Can you work these out from the drawing? Everything is in mm from the part's minimum corner. A direction names the side the tool comes from. Coordinates: 2 decimals unless noted, no trailing zeros. Loops run counter-clockwise (first coordinate to the right, second up) from the corner with the lowest first, then second, coordinate; pieces in that order, holes last. Notation, with made-up numbers: (31, 34) -> (50, 34) arc R22 ccw to (50, 66) -> close; hole circle Ø9 at (21, 88.25). An arc over 180 degrees is marked (long way). One line per question, with ' | ' between items.
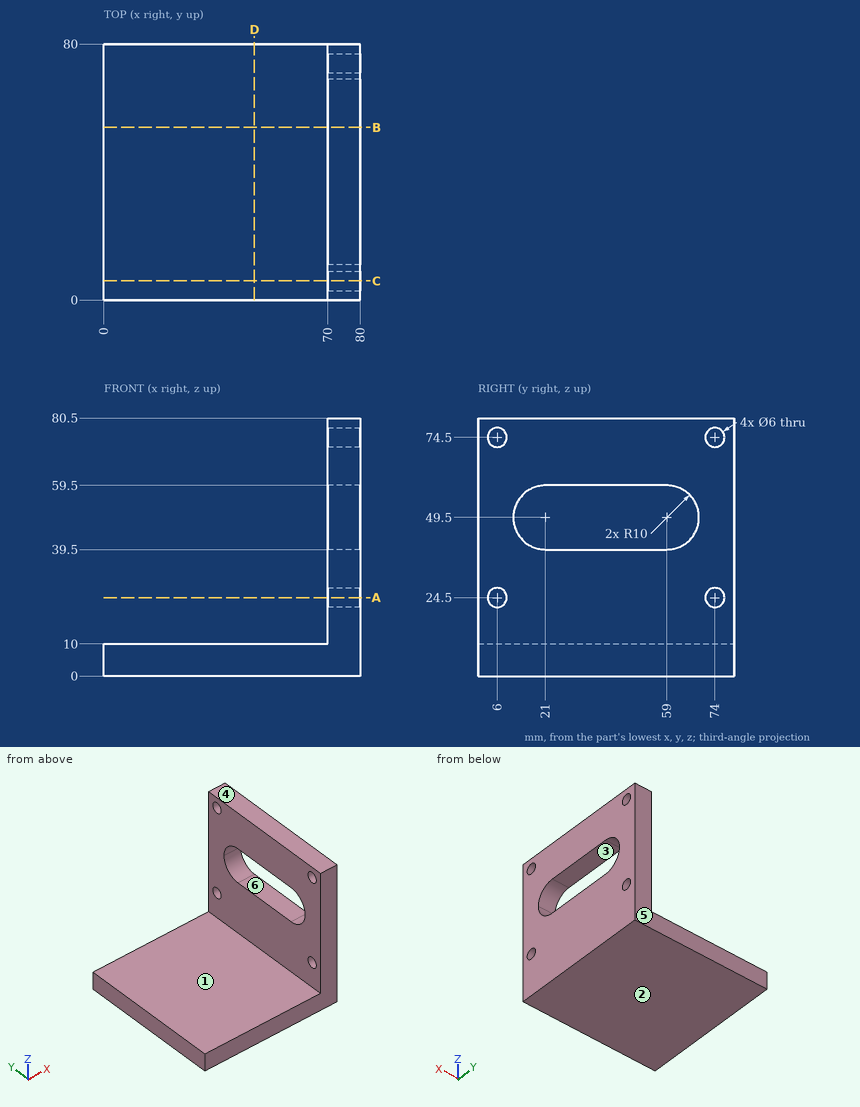
Q1. Please list where these lines run through material, in increasing order: L1, parallel to Y at x = 73, z = 24.5; L2, parallel to Y at x = 72.5, z = 77; L3, parallel to Z at x = 42, y = 50. Write a range as [from, to].
Values follow:
L1: y = [0, 3], [9, 71], [77, 80] | L2: y = [0, 4.34], [7.66, 72.34], [75.66, 80] | L3: z = [0, 10]
Q2. Imagine slicing it at D-D on x = 47. Write out the boundary of the cut face in (y, z).
Values follow:
outline: (0, 0) -> (80, 0) -> (80, 10) -> (0, 10) -> close
Q3. Imagine slicing it at A-A on z = 24.5. Write out the boundary of the cut face in (x, y).
Values follow:
outline: (70, 0) -> (80, 0) -> (80, 3) -> (70, 3) -> close; (70, 9) -> (80, 9) -> (80, 71) -> (70, 71) -> close; (70, 77) -> (80, 77) -> (80, 80) -> (70, 80) -> close
Q4. Imagine slicing it at C-C on y = 6. Write out the boundary of the cut face in (x, z).
Values follow:
outline: (0, 0) -> (80, 0) -> (80, 21.5) -> (70, 21.5) -> (70, 10) -> (0, 10) -> close; (70, 27.5) -> (80, 27.5) -> (80, 71.5) -> (70, 71.5) -> close; (70, 77.5) -> (80, 77.5) -> (80, 80.5) -> (70, 80.5) -> close
Q5. For the marked faces 1, 2 and 3, which set-ups out of +Z, -Z, +X, -X, +Y, -Y let a thin tool reach every point of the face, with its end or its side?
Values follow:
face 1: +Z, -X, +Y, -Y | face 2: -Z, +X, -X, +Y, -Y | face 3: +X, -X
Q6. We'd pull the mould along Y, two halves only. Please class the marked faces 4, 5 and 6: released by +Y, released by -Y, zero draft, split by the parting line, or undercut.
Values follow:
face 4: zero draft | face 5: released by +Y | face 6: undercut
Q7. Imagine slicing it at B-B on y = 54. Write out the boundary of the cut face in (x, z).
Values follow:
outline: (0, 0) -> (80, 0) -> (80, 39.5) -> (70, 39.5) -> (70, 10) -> (0, 10) -> close; (70, 59.5) -> (80, 59.5) -> (80, 80.5) -> (70, 80.5) -> close
Q8. For pin 1 (21 mm diameter, centred on x = 43, y = 35, fed in from +Z); pin 2 (21 mm diameter, centred on y = 40, z = 35.5, fed in from -X), each with a flat end and sliding along its axis, tell me the tip position at first contact or that it passes through.
Values follow:
pin 1: stops at z = 10 | pin 2: stops at x = 70
